```python
from build123d import *

# Parameters (mm, degrees)
SKETCH1_W           = 350
SKETCH1_H           = 140
BOSS_EXTRUDE1_DEPTH = 4
SKETCH2_R           = 2.5
SKETCH2_W           = 42
SKETCH2_H           = 42
CUT_EXTRUDE1_DEPTH  = 5
SKETCH3_R           = 2
CUT_EXTRUDE2_DEPTH  = 10


with BuildPart() as part:
    # Sketch1 → Boss-Extrude1 (new body)
    with BuildSketch(Plane(origin=(0, 0, 0), x_dir=(1, 0, 0), z_dir=(0, 1, 0))):
        Rectangle(SKETCH1_W, SKETCH1_H)
    extrude(amount=BOSS_EXTRUDE1_DEPTH)

    # Sketch2 → Cut-Extrude1 (cut, through all)
    with BuildSketch(Plane(origin=(0, 4, 0), x_dir=(1, 0, 0), z_dir=(0, 1, 0))):
        with Locations((-165, 13)):
            Circle(SKETCH2_R)
        with Locations((-165, -13)):
            Circle(SKETCH2_R)
        with Locations((165, -13)):
            Circle(SKETCH2_R)
        with Locations((165, 13)):
            Circle(SKETCH2_R)
        with Locations((-118, 60)):
            Circle(SKETCH2_R)
        with Locations((-58, 60)):
            Circle(SKETCH2_R)
        with Locations((58, 60)):
            Circle(SKETCH2_R)
        with Locations((118, 60)):
            Circle(SKETCH2_R)
        with Locations((118, -60)):
            Circle(SKETCH2_R)
        with Locations((58, -60)):
            Circle(SKETCH2_R)
        with Locations((-58, -60)):
            Circle(SKETCH2_R)
        with Locations((-118, -60)):
            Circle(SKETCH2_R)
        with Locations((-154, -49)):
            Rectangle(SKETCH2_W, SKETCH2_H)
        with Locations((154, -49)):
            Rectangle(SKETCH2_W, SKETCH2_H)
        with Locations((154, 49)):
            Rectangle(SKETCH2_W, SKETCH2_H)
        with Locations((-154, 49)):
            Rectangle(SKETCH2_W, SKETCH2_H)
    extrude(amount=-CUT_EXTRUDE1_DEPTH, mode=Mode.SUBTRACT)

    # Sketch3 → Cut-Extrude2 (cut)
    with BuildSketch(Plane(origin=(0, 4, 0), x_dir=(1, 0, 0), z_dir=(0, 1, 0))):
        with Locations((-131, -6)):
            Circle(SKETCH3_R)
        with Locations((-101, -6)):
            Circle(SKETCH3_R)
        with Locations((-101, 18)):
            Circle(SKETCH3_R)
        with Locations((101, -6)):
            Circle(SKETCH3_R)
        with Locations((-131, 18)):
            Circle(SKETCH3_R)
        with Locations((101, 18)):
            Circle(SKETCH3_R)
        with Locations((131, 18)):
            Circle(SKETCH3_R)
        with Locations((131, -6)):
            Circle(SKETCH3_R)
    extrude(amount=-CUT_EXTRUDE2_DEPTH, mode=Mode.SUBTRACT)


solid = part.part
```
Design review of the part built by this model. Coordinates are the model's own, in mm. Coordinates: 2 decimals unless noted, no trailing zeros. Write each loop counter-clockwise with the first axis right and the second up, starting at its lowest first coordinate (ties: lowest second). Pieces come first, ordered by that corner, then holes.
1) Insertion check: pin 1 (2.5 mm diameter, centred on x = -101, z = -18, fed in from +Y); pin 2 (1 mm diameter, centred on y = 0.5, z = -39.5, fed in from -X); pin 3 (2 mm diameter, centred on x = 161, y = 2.5, fed in from -Z). Each pin has a flat end and moves straight along its axis. Give the tip position at first contact, or say it passes through.
2) Add section C-C (x = -147.5). Write out the cut boundary in (y, z).
3) To check wall thickness, follow L1, parallel to Z at x = -58, y = 2.3; L2, parallel to Z at x = -165, y = 1.7; L3, parallel to X at y = 2.2, z = -18. State the ranges of each line that lie inside material, in increasing order.
4) Add section B-B (z = 51). Write out the cut boundary in (x, y).
5) Add section A-A (y = 2). State how many separate pieces and enclosed holes the cut face has, plus the area to 3 significant figures.
Check result:
1. pin 1: passes through
1. pin 2: stops at x = -133
1. pin 3: stops at z = -28
2. outline: (0, -28) - (4, -28) - (4, 28) - (0, 28) - close
3. L1: z = -70 to -62.5, -57.5 to 57.5, 62.5 to 70
3. L2: z = -28 to -15.5, -10.5 to 10.5, 15.5 to 28
3. L3: x = -175 to -133, -129 to -103, -99 to 99, 103 to 129, 133 to 175
4. outline: (-133, 0) - (133, 0) - (133, 4) - (-133, 4) - close
5. separate pieces: 1
5. enclosed holes: 20
5. area: 41,600 mm2
